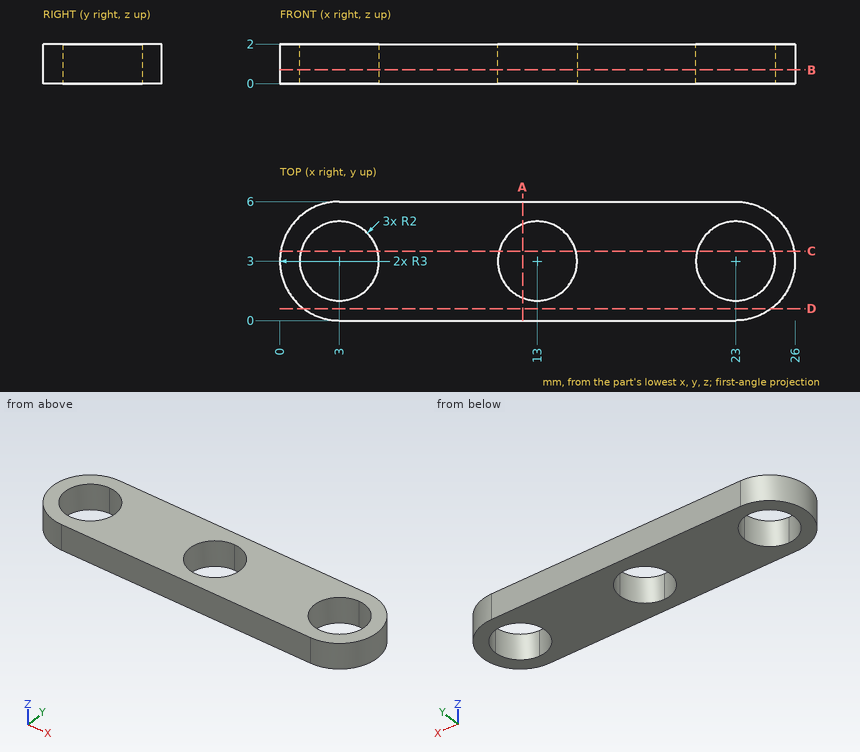
The drawing under review shows one solid part. Ordinate dimensions are in mm from its lowest x, y, z. Give positions to 0.01 mm unless a question says otherwise; leave off trailing zeros. Write each loop counter-clockwise with the first axis right and the second up, starting at its lowest first coordinate (ties: lowest second). Pieces come first, ordered by that corner, then holes. Notation, with made-up numbers: (10, 21) -> (39, 21) arc R29 cw to (39, 46) -> close; hole circle Ø7 at (56, -6). An arc over 180 degrees is marked (long way). Use CSV: the item, a comma, the result in double quotes.
Q1. Take a section at D-D, the plane y = 0.6. Write out the cut boundary in (x, z).
Conclusion:
outline,"(1.2, 0) -> (24.8, 0) -> (24.8, 2) -> (1.2, 2) -> close"
Q2. Take a section at A-A, the plane x = 12.25. Write out the cut boundary in (y, z), then the cut area to 3 significant figures.
Conclusion:
outline,"(0, 0) -> (1.15, 0) -> (1.15, 2) -> (0, 2) -> close; (4.85, 0) -> (6, 0) -> (6, 2) -> (4.85, 2) -> close"
area,"4.58 mm2"
Q3. For P1, Ø1, axis at x = 7.5, z = 1.5, coming from the -Y side, flat-tipped, find the tip position at first contact; note if it passes through.
Conclusion:
P1,"y = 0"
Q4. To check wall thickness, follow probe 1 along X at (y, z) = (3.05, 1.85); probe 2 along X at (y, z) = (2.55, 0.9); probe 3 along Y at (x, z) = (2.5, 0.6). State the ranges of each line that lie inside material, in increasing order. Write a range as [from, to].
Conclusion:
probe 1,"[0, 1], [5, 11], [15, 21], [25, 26]"
probe 2,"[0.03, 1.05], [4.95, 11.05], [14.95, 21.05], [24.95, 25.97]"
probe 3,"[0.04, 1.06], [4.94, 5.96]"
Q5. Take a section at C-C, the plane y = 3.5. Write out the cut boundary in (x, z), then the cut area to 3 significant figures.
Conclusion:
outline,"(0.04, 0) -> (1.06, 0) -> (1.06, 2) -> (0.04, 2) -> close; (4.94, 0) -> (11.06, 0) -> (11.06, 2) -> (4.94, 2) -> close; (14.94, 0) -> (21.06, 0) -> (21.06, 2) -> (14.94, 2) -> close; (24.94, 0) -> (25.96, 0) -> (25.96, 2) -> (24.94, 2) -> close"
area,"28.6 mm2"
Q6. Take a section at B-B, the plane z = 0.7. Write out the cut boundary in (x, y).
Conclusion:
outline,"(3, 0) -> (23, 0) arc R3 ccw to (23, 6) -> (3, 6) arc R3 ccw to start; hole circle Ø4 at (3, 3); hole circle Ø4 at (13, 3); hole circle Ø4 at (23, 3)"
